from build123d import *
from build123d.topology import SkipClean

# Parameters (mm, degrees)
CUT_REVOLVE2_ANGLE      = 180
BOSS_EXTRUDE1_START     = -0.0001
BOSS_EXTRUDE1_OUTLINE_R = 33.75
BOSS_EXTRUDE1_DEPTH     = 3.0001
SKETCH7_R               = 29.5
BOSS_EXTRUDE2_DEPTH     = 12
SKETCH8_R               = 32
BOSS_EXTRUDE3_DEPTH     = 3
SKETCH9_R               = 28
CUT_EXTRUDE1_DEPTH      = 16


# Read off the part's stored shape, not the designer's step: Boss-Extrude1
with BuildPart() as part:
    # Sketch1 → Revolve1 (revolve)
    with BuildSketch(Plane.XY):
        with BuildLine():
            Line((35, 0), (-35, 0))
            ThreePointArc((-35, 0), (0, 35), (35, 0))
        make_face()
    revolve(axis=Axis((35, 0, 0), (-1, 0, 0)))

    # Sketch3 → Cut-Revolve1 (revolve, cut)
    with BuildSketch(Plane.XY):
        with BuildLine():
            Line((0.536808441, 33.745730644), (-0.536808441, -33.745730644))
            ThreePointArc((-0.536808441, -33.745730644), (-33.745730644, 0.536808441), (0.536808441, 33.745730644))
        make_face()
    revolve(axis=Axis((0.536808441, 33.745730644, 0), (-0.015905435294566866, -0.9998735005629914, 0)), mode=Mode.SUBTRACT)

    # Sketch5 → Cut-Revolve2 (revolve, cut)
    with SkipClean():  # the faces are left unmerged after this step: merging them gives an invalid solid
        with BuildSketch(Plane(origin=(0, 0, 0), x_dir=(1, 0, 0), z_dir=(0, 1, 0))):
            with BuildLine():
                Line((-35, 0), (35, 0))
                ThreePointArc((35, 0), (0, -35), (-35, 0))
            make_face()
        revolve(axis=Axis((-35, 0, 0), (1, 0, 0)), revolution_arc=CUT_REVOLVE2_ANGLE, mode=Mode.SUBTRACT)

    # Boss-Extrude1 outline → Boss-Extrude1 (add)
    with SkipClean():  # the faces are left unmerged after this step: merging them gives an invalid solid
        with BuildSketch(Plane(origin=(0, 0, 0), x_dir=(1, 0, 0), z_dir=(0, 1, 0)).offset(BOSS_EXTRUDE1_START)):
            Circle(BOSS_EXTRUDE1_OUTLINE_R)
        extrude(amount=BOSS_EXTRUDE1_DEPTH)

    # Sketch7 → Boss-Extrude2 (add)
    with SkipClean():  # the faces are left unmerged after this step: merging them gives an invalid solid
        with BuildSketch(Plane.XZ.offset(0.0001)):
            with Locations(Location((0, 0, 0), (0, 0, 270))):
                Circle(SKETCH7_R)
        extrude(amount=BOSS_EXTRUDE2_DEPTH)

    # Sketch8 → Boss-Extrude3 (add)
    with SkipClean():  # the faces are left unmerged after this step: merging them gives an invalid solid
        with BuildSketch(Plane.XZ.offset(12.0001)):
            with Locations(Location((0, 0, 0), (0, 0, 270))):
                Circle(SKETCH8_R)
        extrude(amount=-BOSS_EXTRUDE3_DEPTH)

    # Sketch9 → Cut-Extrude1 (cut)
    with SkipClean():  # the faces are left unmerged after this step: merging them gives an invalid solid
        with BuildSketch(Plane.XZ.offset(12.0001)):
            with Locations(Location((0, 0, 0), (0, 0, 270))):
                Circle(SKETCH9_R)
        extrude(amount=-CUT_EXTRUDE1_DEPTH, mode=Mode.SUBTRACT)


solid = part.part
Work out the finished part from the listing and answer in its coordinate system (mm). A direction names the side the tool comes from. Round coordinates to 2 decimals unless told otherwise and drop trailing zeros. Write each loop counter-clockwise with the first axis right and the second up, starting at its lowest first coordinate (ties: lowest second). Pieces come first, ordered by that corner, then holes. Notation, with made-up numbers: M 5.5,68 L 28.5,68 A20 ccw 28.5,104 Z; hole C -6,50 d11. An arc over 180 degrees is marked long. Use a Markdown table: item, result.
1) Consider line 1 (X direction, y = -2.75, z = 0); line 2 (Y direction, x = 29.5, z = -2.5); line 3 (X direction, y = 23, z = 7). Determine where each line is inside the solid, lowest interval first. Write a range as [from, to].
Taken from the geometry:
| item | result |
|---|---|
| line 1 | x = [-29.5, -28], [28, 29.5] |
| line 2 | y = [-12, -9], [0, 3], [16.2, 18.67] |
| line 3 | x = [-25.44, -23.69], [23.69, 25.44] |
2) Determine the mould class of faces 3 (the face through (7, -9, 29)), 4 (the face through (-13, 3, -25)), 5 (the face through (8.86, -4.44, -28.14)) for opening direction Z: pulls with the +Z half, pulls with the -Z half, needs draft (parallel to the pull), parting line crosses it, or undercut.
Taken from the geometry:
| item | result |
|---|---|
| face 3 | needs draft |
| face 4 | undercut |
| face 5 | parting line crosses it |
3) The part is cut by section D-D on y = -2. Give the vertices of the cut face in (x, z).
Taken from the geometry:
| item | result |
|---|---|
| outline | C 0,0 d59; hole C 0,0 d56 |
4) The part is cut by section C-C on y = 11.5. Give the vertices of the cut face in (x, z).
Taken from the geometry:
| item | result |
|---|---|
| outline | C 0,0 d66.11; hole C 0,0 d63.46 |
5) Flat-ended cylindrical pins translate along their axes: pin 1 (10.5 mm diameter, centred on x = -14, z = -14, fed in from -Y); pin 2 (3 mm diameter, centred on y = 19.5, z = 16, fed in from -X); pin 3 (12 mm diameter, centred on x = 26, y = 0, fed in from -Z). Find the tip coordinate at first contact, or state that the pin passes through.
Taken from the geometry:
| item | result |
|---|---|
| pin 1 | stops at y = 22.62 |
| pin 2 | stops at x = -25.73 |
| pin 3 | stops at z = -28.72 |
6) Which of the six approach directions +Z, -Z, +X, -X, +Y, -Y give full straight-line access (tool end or side, diameter ignored) to faces 1 (the face through (0, 0, 30)), 2 (the face through (-31.24, -10.52, 6.94))?
Taken from the geometry:
| item | result |
|---|---|
| face 1 | none |
| face 2 | -Y |
